Could you check a few things on this model? Use its own coordinates, in mm. A direction names the side the tool comes from. Coordinates: 2 decimals unless noted, no trailing zeros. Loops run counter-clockwise (first coordinate to the right, second up) from the corner with the lowest first, then second, coordinate; pieces in that order, holes last. Notation, with made-up numbers: M 2.25,-24.5 L 25.25,-24.5 A29 ccw 25.25,1.5 Z; hole C 31.25,51 d10. An arc over 180 degrees is marked long. Write each question's results on one line, items separated by ' | '.
Autodesk Inventor part; units mm, degrees
ref_plane "YZ Plane" through (0, 0, 0) normal (1, 0, 0) x (0, 1, 0)
ref_plane "XZ Plane" through (0, 0, 0) normal (0, 1, 0) x (-1, 0, 0)
ref_plane "XY Plane" through (0, 0, 0) normal (0, 0, 1) x (1, 0, 0)
sketch "Sketch2" plane through (-15, -30, 0) normal (0, 0, 1) x (1, 0, 0)
  arc A0 (22.5, 30) -> (7.5, 30) centre (15, 30) ccw
  line L0 (7.5, 30) -> (0, 10)
  line L1 (30, 10) -> (22.5, 30)
  line L2 (30, 0) -> (30, 10)
  line L3 (0, 10) -> (0, 0)
  line L4 (0, 0) -> (30, 0)
  circle A1 centre (15, 30) radius 2.75
  circle A2 centre (15, 8) radius 1.7
  line L5 (15, 30) -> (15, 8) construction
  line L6 (7.5, 30) -> (15, 30) construction
  dimension "d15" = 30
  dimension "d16" = 10
  dimension "d17" = 15
  dimension "d18" = 5.5
  dimension "d19" = 30
  dimension "d20" = 8
  dimension "d21" = 15
  dimension "d22" = 3.4
extrude "Extrusion1" add sketch "Sketch2" along normal blind 2
sketch "Sketch3" plane through (-15, -30, 0) normal (0, -1, 0) x (1, 0, 0)
  line L0 (0, 0) -> (30, 0)
  line L1 (30, 0) -> (30, 2)
  line L2 (0, 2) -> (30, 2)
  line L3 (0, 0) -> (0, 2)
  point P0 (15, 0)
extrude "Extrusion2" add sketch "Sketch3" along normal blind 3.5
sketch "Sketch4" plane through (-15, -30, 0) normal (0, 0, -1) x (-1, 0, 0)
  line L0 (-30, 10) -> (-30, -3.5)
  line L1 (0, 10) -> (0, -3.5)
  line L2 (-30, -3.5) -> (0, -3.5)
  line L3 (0, -3.5) -> (0, -1.5)
  line L4 (0, -1.5) -> (-30, -1.5)
  line L5 (-30, -1.5) -> (-30, -3.5)
  point P0 (-15, 30)
  dimension "d27" = 2
extrude "Extrusion3" add sketch "Sketch4" along normal blind 19
sketch "Sketch5" plane through (-15, -33.5, 0) normal (0, -1, 0) x (1, 0, 0)
  line L0 (10, -4.5) -> (20, -4.5)
  line L1 (20, -4.5) -> (20, -14.5)
  line L2 (20, -14.5) -> (10, -14.5)
  line L3 (10, -14.5) -> (10, -4.5)
  line L4 (10, -4.5) -> (20, -14.5) construction
  line L5 (20, -4.5) -> (10, -14.5) construction
  line L6 (15, 0) -> (15, -9.5) construction
  line L7 (30, 0) -> (0, 0)
  line L8 (30, -19) -> (0, -19)
  dimension "d31" = 10
  dimension "d32" = 9.5
  dimension "d33" = 10
extrude "Extrusion4" cut sketch "Sketch5" against normal up to next
sketch "Sketch6" plane through (-15, -31.5, 0) normal (0, 1, 0) x (1, 0, 0)
  line L0 (20, 4.5) -> (10, 4.5)
  line L1 (20, 14.5) -> (20, 4.5)
  line L2 (10, 4.5) -> (10, 14.5)
  line L3 (10, 14.5) -> (20, 14.5)
  line L4 (21.5, 3) -> (8.5, 3)
  line L5 (8.5, 3) -> (8.5, 16)
  line L6 (8.5, 16) -> (21.5, 16)
  line L7 (21.5, 16) -> (21.5, 3)
  point P0 (15, 0)
  dimension "d36" = 1.5
extrude "Extrusion5" add sketch "Sketch6" along normal blind 1.5
sketch "Sketch7" plane through (-15, -30, 2) normal (0, 0, 1) x (1, 0, 0)
  circle A0 centre (15, 30) radius 4.275
  dimension "d39" = 8.55
extrude "Extrusion6" cut sketch "Sketch7" against normal blind 0.1
properties part number "LampeSolaire2_LedAmoviblePart_Cover 3D printer"
(1) Which directions (+Z, -Z, +X, -X, +Y, -Y) give clear straight access to the entire face, cutting with the end or side of a thin tool? Please do faces 1 (the flat face through (-5, -32, -9)), 2 (the flat face through (0, -31, -3)), 3 (the flat face through (6.5, -31, -10)), 4 (the flat face through (0, -31, -16)).
Reported:
face 1: +Y, -Y | face 2: +X, -X, +Y | face 3: -Z, +X, +Y | face 4: -Z, +X, -X, +Y
(2) Imagine slicing it at D-D, the plane z = -4. List the corners of the cut face in (x, y) for me.
Reported:
outline: M -15,-33.5 L 15,-33.5 L 15,-31.5 L 6.5,-31.5 L 6.5,-30 L -6.5,-30 L -6.5,-31.5 L -15,-31.5 Z
(3) Please list where these lines run through material, in increasing order: probe 1 along Y at (x, z) = (0, 1.25); probe 2 along X at (y, z) = (0, 1.55); probe 3 along Z at (x, y) = (-6, -15). Write a range as from..to.
Reported:
probe 1: y = -33.5..-23.7, -20.3..-2.75, 2.75..7.5 | probe 2: x = -7.5..-2.75, 2.75..7.5 | probe 3: z = 0..2
(4) Imagine slicing it at C-C, the plane z = -10.5. List the corners of the cut face in (x, y) for me, and give its area (3 significant figures).
Reported:
outline: M -15,-33.5 L -5,-33.5 L -5,-30 L -6.5,-30 L -6.5,-31.5 L -15,-31.5 Z; M 5,-33.5 L 15,-33.5 L 15,-31.5 L 6.5,-31.5 L 6.5,-30 L 5,-30 Z | area: 44.5 mm2
(5) If we mould it in two halves opening along Z, with no side actions, what happens to faces 5 (the flat face through (0, -32, -14.5)), 6 (the cylindrical face through (-0.16, 7.5, 0.99)), 7 (the flat face through (0, -32, -19)), 8 (the flat face through (0, -32, -4.5))? For each: released by +Z, released by -Z, zero draft, split by the parting line, or undercut.
Reported:
face 5: undercut | face 6: zero draft | face 7: released by -Z | face 8: undercut
(6) Imagine slicing it at B-B, the plane x = 0. List the corners of the cut face in (y, z) for me (3 decimals), and give its area (3 significant figures).
Reported:
outline: M -33.5,-19 L -31.5,-19 L -31.5,-16 L -30,-16 L -30,-14.5 L -33.5,-14.5 Z; M -33.5,-4.5 L -30,-4.5 L -30,-3 L -31.5,-3 L -31.5,0 L -23.7,0 L -23.7,2 L -33.5,2 Z; M -20.3,0 L -2.75,0 L -2.75,1.9 L -4.275,1.9 L -4.275,2 L -20.3,2 Z; M 2.75,0 L 7.5,0 L 7.5,2 L 4.275,2 L 4.275,1.9 L 2.75,1.9 Z | area: 86.4 mm2
(7) Will these pins go through, and if not, where does the flat tip stop? P1, Ø5, axis at x = 2, y = -1, coming from the -Z side; P2, Ø0.8, axis at y = -31, z = -9, coming from the -X side; P3, Ø0.8, axis at x = 0.5, y = -30.5, coming from the -Z side.
Reported:
P1: stops at z = 0 | P2: stops at x = -6.5 | P3: stops at z = -16
(8) Imagine slicing it at A-A, the plane y = -22. List the corners of the cut face in (x, z) for me, and give its area (3 significant figures).
Reported:
outline: M -15,0 L -1.7,0 L -1.7,2 L -15,2 Z; M 1.7,0 L 15,0 L 15,2 L 1.7,2 Z | area: 53.2 mm2
